```python
from build123d import *

# Parameters (mm, degrees)
F0_W     = 8.75
F0_H     = 7.5
F1_DEPTH = 8
F1_TAPER = 1
F2_W     = 8.7793770789
F2_H     = 14
F3_DEPTH = 2
F4_R     = 1


with BuildPart() as f1:
    # F0 (on Top) → F1 (new body)
    with BuildSketch(Plane.XY):
        Rectangle(F0_W, F0_H)
    extrude(amount=F1_DEPTH, taper=F1_TAPER)

    # F2 (on face) → F3 (join)
    with BuildSketch(Plane(origin=(0, 0, 0), x_dir=(1, 0, 0), z_dir=(0, 0, -1))):
        Rectangle(F2_W, F2_H)
    extrude(amount=F3_DEPTH)

    # F4
    f4_edges = [f1.edges().sort_by_distance(p)[0] for p in [
        (0, -3.610359, 8),
        (4.235359, 0, 8),
        (0, 3.610359, 8),
        (-4.235359, 0, 8),
        (4.30518, -3.68018, 4),
        (-4.30518, -3.68018, 4),
        (-4.30518, 3.68018, 4),
        (4.30518, 3.68018, 4),
        (4.389689, -7, -1),
        (-4.389689, -7, -1),
        (4.389689, 7, -1),
        (-4.389689, 7, -1),
    ]]
    fillet(f4_edges, radius=F4_R)


solid = f1.part
```
CAD build for the part. Positions are in the model's coordinates, mm. A direction names the side the tool comes from. Round coordinates to 2 decimals unless told otherwise and drop trailing zeros. Loops run counter-clockwise (first coordinate to the right, second up) from the corner with the lowest first, then second, coordinate; pieces in that order, holes last. Notation, with made-up numbers: (-38, -4) - (-14, -4) arc R31 ccw to (-14, 35) - close; hole circle Ø6 at (55.25, -33.75). An arc over 180 degrees is marked (long way). Return JSON: item names as keys, results as strings. Group by question number.
Q1. Band-saw the part on A-A on x = 1. Give the cut face in (y, z), plus the area to 3 significant figures.
Q2. Drill centre lines: line 1 along Z through (x, y) = (-2.75, -4.75); line 2 along Y through (x, z) = (-2.75, 0.25); line 3 along X through (y, z) = (-1.75, 0.25). Where is each one in solid material? Low to high. Write a range as [from, to].
Q3. Band-saw the part on C-C on y = -4.75. Give the cut face in (x, z), plus the area to 3 significant figures.
Q4. Tool access for faces 1 (the face through (-4.028, 3.387, 3.56)), 2 (the face through (-4.028, -3.387, 3.56)), 3 (the face through (0.046, -3.336, 7.706)), 4 (the face through (4.012, 3.403, 3.56)): list every direction of +Z, -Z, +X, -X, +Y, -Y with a clear straight run to the whole face (end or side of a thin tool).
Q5. Flat gauge pins, fed straight in: pin 1 Ø6 at (y, z) = (-1.5, 7) entering from -X; pin 2 Ø1 at (x, z) = (2, 4) entering from -Y. Where does each tip first touch, or does it go through?
Solutions:
{
 "1": {"outline": "(-7, -2) - (7, -2) - (7, 0) - (3.75, 0) - (3.63, 7.02) arc R1 ccw to (2.63, 8) - (-2.63, 8) arc R1 ccw to (-3.63, 7.02) - (-3.75, 0) - (-7, 0) - close", "area": "86.5 mm^2"},
 "2": {"line 1": "z = [-2, 0]", "line 2": "y = [-3.75, 3.75]", "line 3": "x = [-4.37, 4.37]"},
 "3": {"outline": "(-4.39, -2) - (4.39, -2) - (4.39, 0) - (-4.39, 0) - close", "area": "17.6 mm^2"},
 "4": {"face 1": "+Z, -X, +Y", "face 2": "+Z, -X, -Y", "face 3": "+Z, +X, -X, -Y", "face 4": "+Z, +X, +Y"},
 "5": {"pin 1": "stops at x = -4.31", "pin 2": "stops at y = -3.69"}
}
